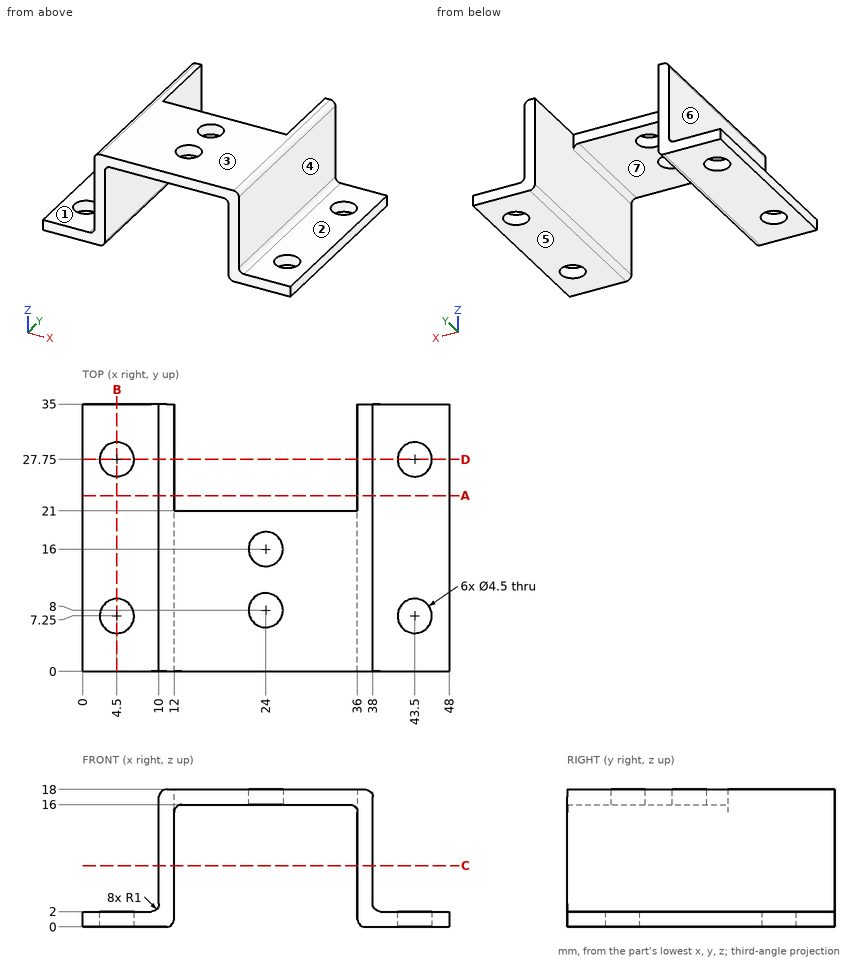
Part print with two shaded views. Sizes in mm from the minimum x, y, z corner. A direction names the side the tool comes from. Coordinates: 2 decimals unless noted, no trailing zeros. Loops run counter-clockwise (first coordinate to the right, second up) from the corner with the lowest first, then second, coordinate; pieces in that order, holes last. Notation, with made-up numbers: M 89,-36 L 141,-36 A19 ccw 141,-22 Z; hole C 30.5,69 d9. An arc over 180 degrees is marked long. Use CSV: the item, a comma, the result in double quotes. Start each with the question number.
1. Probe probe 1 along Y at (x, z) = (24, 17.5); probe 2 along Y at (x, z) = (43.5, 0.7); probe 3 along X at (y, z) = (29, 12.5). List the from-to ranges inside material, lowest first. Write a range as [from, to].
2. Band-saw the part on C-C, the plane z = 8. List the corners of the cut face in (x, y), then the cut area to 3 significant figures.
3. Two-plate mould, pull along X, no slides. Class the marked faces 4, 5, 6 and 7: pulls with the +X half, pulls with the -X half, needs draft (parallel to the pull), parting line crosses it, or undercut.
4. Band-saw the part on A-A, the plane y = 23. List the corners of the cut face in (x, z), then the cut area to 3 significant figures.
5. Band-saw the part on D-D, the plane y = 27.75. List the corners of the cut face in (x, z), then the cut area to 3 significant figures.
6. Band-saw the part on B-B, the plane x = 4.5. List the corners of the cut face in (y, z).
7. Flat gauge pins, fed straight in: pin 1 (8.5 mm diameter, centred on y = 20.5, z = 9, fed in from +X); pin 2 (5 mm diameter, centred on x = 24, y = 16, fed in from -Z); pin 3 (4.5 mm diameter, centred on x = 3.5, y = 14.5, fed in from +Z). Where does each tip first touch, or does it go through?
8. Tool access for the marked faces 1, 2 and 3: list every direction of +Z, -Z, +X, -X, +Y, -Y with a clear straight run to the whole face (end or side of a thin tool).
Entries:
1,probe 1,"y = [0, 5.75], [10.25, 13.75], [18.25, 21]"
1,probe 2,"y = [0, 5], [9.5, 25.5], [30, 35]"
1,probe 3,"x = [10, 12], [36, 38]"
2,outline,"M 10,0 L 12,0 L 12,35 L 10,35 Z; M 36,0 L 38,0 L 38,35 L 36,35 Z"
2,area,"140 mm2"
3,face 4,"pulls with the +X half"
3,face 5,"needs draft"
3,face 6,"pulls with the -X half"
3,face 7,"undercut"
4,outline,"M 0,0 L 11,0 A1 ccw 12,1 L 12,18 L 11,18 A1 ccw 10,17 L 10,3 A1 cw 9,2 L 0,2 Z; M 36,1 A1 ccw 37,0 L 48,0 L 48,2 L 39,2 A1 cw 38,3 L 38,17 A1 ccw 37,18 L 36,18 Z"
4,area,"112 mm2"
5,outline,"M 0,0 L 2.25,0 L 2.25,2 L 0,2 Z; M 6.75,0 L 11,0 A1 ccw 12,1 L 12,18 L 11,18 A1 ccw 10,17 L 10,3 A1 cw 9,2 L 6.75,2 Z; M 36,1 A1 ccw 37,0 L 41.25,0 L 41.25,2 L 39,2 A1 cw 38,3 L 38,17 A1 ccw 37,18 L 36,18 Z; M 45.75,0 L 48,0 L 48,2 L 45.75,2 Z"
5,area,"93.6 mm2"
6,outline,"M 0,0 L 5,0 L 5,2 L 0,2 Z; M 9.5,0 L 25.5,0 L 25.5,2 L 9.5,2 Z; M 30,0 L 35,0 L 35,2 L 30,2 Z"
7,pin 1,"stops at x = 38"
7,pin 2,"stops at z = 16"
7,pin 3,"stops at z = 2"
8,face 1,"+Z, -X, +Y, -Y"
8,face 2,"+Z, +X, +Y, -Y"
8,face 3,"+Z, +X, -X, +Y, -Y"
